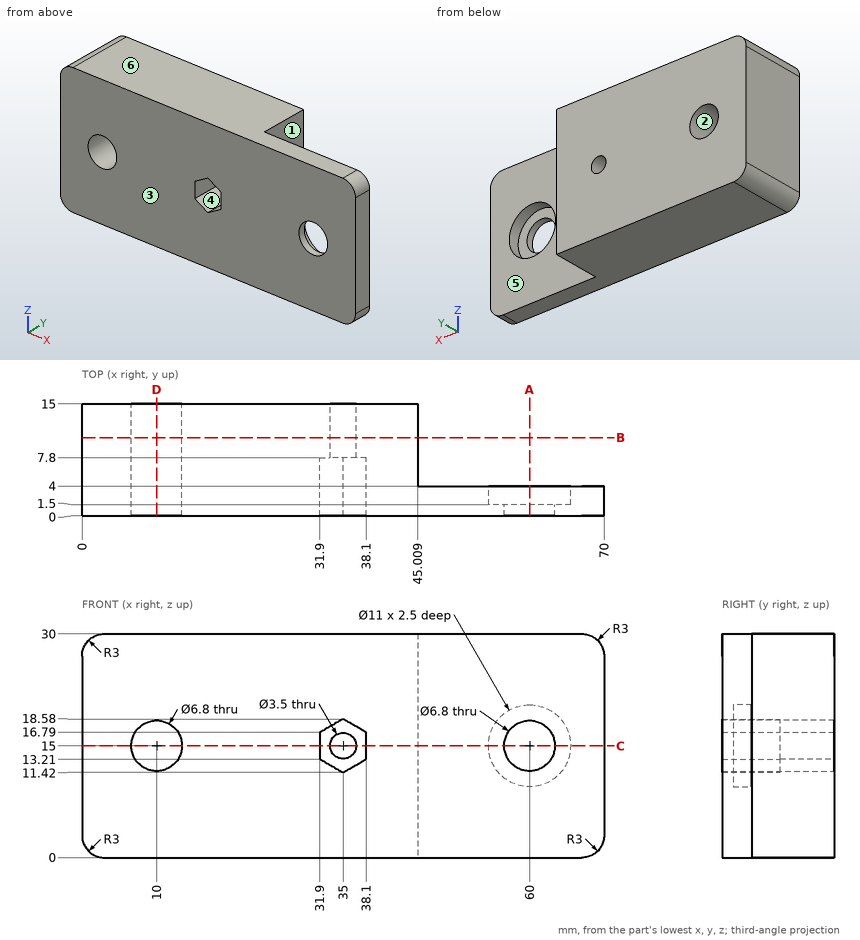
Job drawing, mm, ordinate dimensions from the low corner. One solid piece. A direction names the side the tool comes from. Coordinates: 2 decimals unless noted, no trailing zeros. Loops run counter-clockwise (first coordinate to the right, second up) from the corner with the lowest first, then second, coordinate; pieces in that order, holes last. Notation, with made-up numbers: (80.25, 34) - (122.25, 34) arc R16 cw to (122.25, 46) - close; hole circle Ø6 at (77.5, 39). An arc over 180 degrees is marked (long way). Answer as a JSON object with one key per item and string values. Group by question number.
(1) Cut at B-B (y = 10.5). Give the cut face in (x, z).
(2) Tool access for the marked faces 5 and 6: list every direction of +Z, -Z, +X, -X, +Y, -Y with a clear straight run to the whole face (end or side of a thin tool).
(3) Flat gauge pins, fed straight in: pin 1 (5 mm diameter, centred on x = 35, z = 15, fed in from -Y); pin 2 (17.5 mm diameter, centred on x = 60, z = 15, fed in from +Y). Where does each tip first touch, or does it go through?
(4) Cut at A-A (x = 60). Give the cut face in (y, z).
(5) Probe line 1 along X through (y, z) = (2.35, 15); line 2 along X through (y, z) = (1.1, 15); line 3 along X through (y, z) = (5.5, 17.5) (1 decimal). List the from-to ranges inside material, lowest first.
(6) Cut at D-D (x = 10). Give the cut face in (y, z).
(7) Two-plate mould, pull along X, no slides. Class the marked faces 1, 2, 3 and 4: released by +X, released by -X, zero draft, split by the parting line, or undercut.
(8) Cut at C-C (z = 15). Give the cut face in (x, y), then the cut area to 3 significant figures.
Geometry says:
{
 "1": {"outline": "(0, 3) arc R3 ccw to (3, 0) - (45.01, 0) - (45.01, 30) - (3, 30) arc R3 ccw to (0, 27) - close; hole circle Ø6.8 at (10, 15); hole circle Ø3.5 at (35, 15)"},
 "2": {"face 5": "+Z, -Z, +X, +Y", "face 6": "+Z, +X, -X, +Y, -Y"},
 "3": {"pin 1": "stops at y = 7.8", "pin 2": "stops at y = 4"},
 "4": {"outline": "(0, 0) - (4, 0) - (4, 9.5) - (1.5, 9.5) - (1.5, 11.6) - (0, 11.6) - close; (0, 18.4) - (1.5, 18.4) - (1.5, 20.5) - (4, 20.5) - (4, 30) - (0, 30) - close"},
 "5": {"line 1": "x = 0 to 6.6, 13.4 to 31.9, 38.1 to 54.5, 65.5 to 70", "line 2": "x = 0 to 6.6, 13.4 to 31.9, 38.1 to 56.6, 63.4 to 70", "line 3": "x = 0 to 7.7, 12.3 to 33.1, 36.9 to 45"},
 "6": {"outline": "(0, 0) - (15, 0) - (15, 11.6) - (0, 11.6) - close; (0, 18.4) - (15, 18.4) - (15, 30) - (0, 30) - close"},
 "7": {"face 1": "released by +X", "face 2": "undercut", "face 3": "zero draft", "face 4": "undercut"},
 "8": {"outline": "(0, 0) - (6.6, 0) - (6.6, 15) - (0, 15) - close; (13.4, 0) - (31.9, 0) - (31.9, 7.8) - (33.25, 7.8) - (33.25, 15) - (13.4, 15) - close; (36.75, 7.8) - (38.1, 7.8) - (38.1, 0) - (56.6, 0) - (56.6, 1.5) - (54.5, 1.5) - (54.5, 4) - (45.01, 4) - (45.01, 15) - (36.75, 15) - close; (63.4, 0) - (70, 0) - (70, 4) - (65.5, 4) - (65.5, 1.5) - (63.4, 1.5) - close", "area": "562 mm^2"}
}
